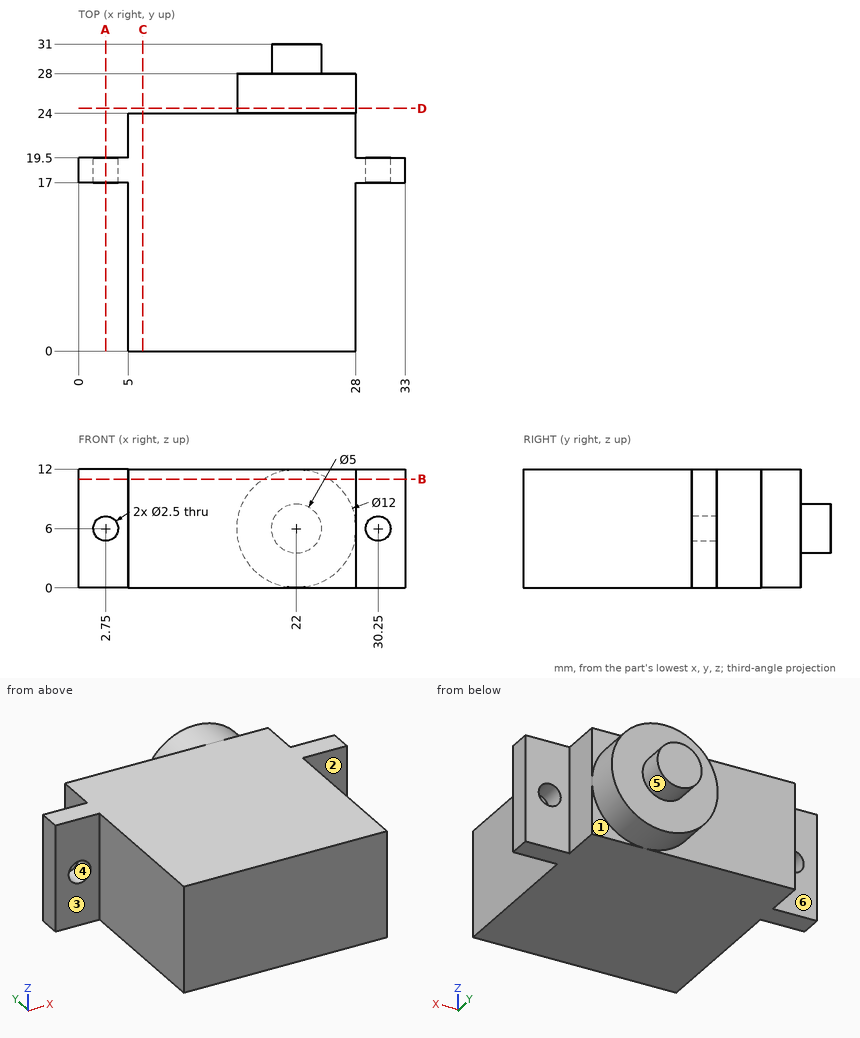
Could you check a few things on this drawing? It's one solid part, dimensions in mm from its lowest x, y, z. A direction names the side the tool comes from. Give positions to 0.01 mm unless a question says otherwise; leave off trailing zeros. Loops run counter-clockwise (first coordinate to the right, second up) from the corner with the lowest first, then second, coordinate; pieces in that order, holes last. Notation, with made-up numbers: (1.5, 89) -> (46.5, 89) arc R19 cw to (46.5, 104) -> close; hole circle Ø4 at (20.25, 21.25). An arc over 180 degrees is marked (long way). Use one line per item in the form item = value. Start each with the question number.
1) Imagine slicing it at A-A (x = 2.75). Please give me the cut outline in (y, z), then the cut area to 4 significant figures.
2) Imagine slicing it at C-C (x = 6.5). Please give me the cut outline in (y, z).
3) Thinking about a two-plate mould opening in Z: for the marked faces 4, 5 and 6, which applies, +Z half, -Z half, draft (parallel to the pull), parting line (faces both ways), or undercut?
4) Imagine slicing it at B-B (z = 11). Please give me the cut outline in (x, y), then the cut area to 3 significant figures.
5) Imagine slicing it at D-D (y = 24.5). Please give me the cut outline in (x, z), then the cut area to 3 significant figures.
6) Which directions (+Z, -Z, +X, -X, +Y, -Y) give clear straight access to the entire face, cutting with the end or side of a thin tool? Please do the marked faces 1, 2 and 3.
7) Please list where these lines run through material, in increasing order: line 1 along X through (y, z) = (17.5, 6); line 2 along Y through (x, z) = (21.5, 0.5); line 3 along X through (y, z) = (4, 8).
8) For P1, Ø6, axis at x = 29, y = 18, coming from the -Z side; P2, Ø2.5, axis at x = 3, z = 4, coming from the -Y side; P3, Ø3, axis at x = 25, z = 2.5, coming from the +Y side; P4, Ø2.5, axis at x = 30, z = 7, coming from the +Y side, each with a flat end and sliding along its axis, tell me the tip position at first contact or that it passes through.
Check values:
q1.outline = (17, 0) -> (19.5, 0) -> (19.5, 4.75) -> (17, 4.75) -> close; (17, 7.25) -> (19.5, 7.25) -> (19.5, 12) -> (17, 12) -> close
q1.area = 23.75 mm^2
q2.outline = (0, 0) -> (24, 0) -> (24, 12) -> (0, 12) -> close
q3.face_4 = undercut
q3.face_5 = parting line
q3.face_6 = draft
q4.outline = (0, 17) -> (5, 17) -> (5, 0) -> (28, 0) -> (28, 17) -> (33, 17) -> (33, 19.5) -> (28, 19.5) -> (28, 24) -> (25.32, 24) -> (25.32, 28) -> (18.68, 28) -> (18.68, 24) -> (5, 24) -> (5, 19.5) -> (0, 19.5) -> close
q4.area = 604 mm^2
q5.outline = circle Ø12 at (22, 6)
q5.area = 113 mm^2
q6.face_1 = -Z, +X, +Y
q6.face_2 = +Z, -Z, +X, -Y
q6.face_3 = +Z, -Z, -X, -Y
q7.line_1 = 0 to 1.5, 4 to 29, 31.5 to 33
q7.line_2 = 0 to 28
q7.line_3 = 5 to 28
q8.P1 = 0
q8.P2 = 17
q8.P3 = 28
q8.P4 = 19.5
